Input: part model. Units: mm. Frame: model coordinates. A direction names the side the tool comes from. Coordinates: 2 decimals unless noted, no trailing zeros. Loops run counter-clockwise (first coordinate to the right, second up) from the corner with the lowest first, then second, coordinate; pieces in that order, holes last. Notation, with made-up numbers: (-0.75, 47) -> (7.25, 47) arc R22 ccw to (7.25, 72) -> close; hole circle Ø10 at (-1, 71). An arc over 180 degrees is marked (long way). Answer as a JSON object with one key per item and string values.
Autodesk Inventor part; units mm, degrees
ref_plane "YZ Plane" through (0, 0, 0) normal (1, 0, 0) x (0, 1, 0)
ref_plane "XZ Plane" through (0, 0, 0) normal (0, 1, 0) x (-1, 0, 0)
ref_plane "XY Plane" through (0, 0, 0) normal (0, 0, 1) x (1, 0, 0)
sketch "Sketch1" plane through (0, 0, 0) normal (0, 0, 1) x (1, 0, 0)
  circle A0 centre (0, 0) radius 120
  circle A1 centre (0, 0) radius 18
  dimension "d0" = 240
  dimension "d1" = 36
extrude "Extrusion1" add sketch "Sketch1" along normal blind 15
sketch "Sketch2" plane through (0, 0, 15) normal (0, 0, 1) x (1, 0, 0)
  circle A0 centre (79.5, 0) radius 23.5
  circle A1 centre (0, 79.5) radius 23.5
  circle A2 centre (-79.5, 0) radius 23.5
  circle A3 centre (0, -79.5) radius 23.5
  point P0 (0, 0)
  dimension "d5" = 47
  dimension "d7" = 47
  dimension "d8" = 47
  dimension "d9" = 47
extrude "Extrusion2" cut sketch "Sketch2" against normal blind 12
sketch "Sketch3" plane through (0, 0, 15) normal (0, 0, 1) x (1, 0, 0)
  circle A0 centre (0, 0) radius 21
  dimension "d12" = 42
extrude "Extrusion3" cut sketch "Sketch3" against normal blind 12
sketch "Sketch4" plane through (0, 0, 15) normal (0, 0, 1) x (1, 0, 0)
  circle A0 centre (0, 0) radius 18
  circle A1 centre (0, 0) radius 119
  circle A2 centre (0, 0) radius 120
  dimension "d15" = 238
  dimension "d16" = 240
extrude "Extrusion4" cut sketch "Sketch4" against normal blind 2 contours A2
sketch "Sketch5" plane through (0, 0, 15) normal (0, 0, 1) x (1, 0, 0)
  circle A0 centre (0, 0) radius 21
  line L0 (0, 0) -> (0, 113.556) construction
  circle A1 centre (0, 113.556) radius 2.5
  circle A2 centre (0, 0) radius 18
  circle A3 centre (0, 0) radius 113.556
  circle A4 centre (-66.7465, 91.8687) radius 2.5
  circle A5 centre (-107.9982, 35.0907) radius 2.5
  circle A6 centre (-107.9982, -35.0907) radius 2.5
  circle A7 centre (-66.7465, -91.8687) radius 2.5
  circle A8 centre (0, -113.556) radius 2.5
  circle A9 centre (66.7465, -91.8687) radius 2.5
  circle A10 centre (107.9982, -35.0907) radius 2.5
  circle A11 centre (107.9982, 35.0907) radius 2.5
  circle A12 centre (66.7465, 91.8687) radius 2.5
  dimension "d19" = 113.556
  dimension "d20" = 5
  dimension "d24" = 360
extrude "Extrusion5" cut sketch "Sketch5" against normal blind 15 contours A1 A3 | A3 A1 | A4 A3 | A3 A4 | A12 A3 | A3 A12 | A5 A3 | A3 A5 | A11 A3 | A3 A11 | A6 A3 | A3 A6 | A10 A3 | A3 A10 | A7 A3 | A3 A7 | A9 A3 | A3 A9 | A8 A3 | A3 A8
sketch "Sketch7" plane through (0, 0, 0) normal (0, 0, -1) x (-1, 0, 0)
  circle A0 centre (0, 113.556) radius 2.5
  circle A1 centre (0, 113.556) radius 6.12
  circle A2 centre (0, 0) radius 113.556 construction
  circle A3 centre (0, 0) radius 113.556 construction
  circle A4 centre (-66.7465, 91.8687) radius 6.12
  circle A5 centre (0, 0) radius 113.556 construction
  circle A6 centre (-107.9982, 35.0907) radius 6.12
  circle A7 centre (0, 0) radius 113.556 construction
  circle A8 centre (-107.9982, -35.0907) radius 6.12
  circle A9 centre (0, 0) radius 113.556 construction
  circle A10 centre (-66.7465, -91.8687) radius 6.12
  circle A11 centre (0, 0) radius 113.556 construction
  circle A12 centre (0, -113.556) radius 6.12
  circle A13 centre (0, 0) radius 113.556 construction
  circle A14 centre (66.7465, -91.8687) radius 6.12
  circle A15 centre (0, 0) radius 113.556 construction
  circle A16 centre (107.9982, -35.0907) radius 6.12
  circle A17 centre (0, 0) radius 113.556 construction
  circle A18 centre (107.9982, 35.0907) radius 6.12
  circle A19 centre (0, 0) radius 113.556 construction
  circle A20 centre (66.7465, 91.8687) radius 6.12
  dimension "d28" = 12.24
  dimension "d31" = 360
extrude "Extrusion6" cut sketch "Sketch7" against normal blind 2 contours A0 | A1 | A4 | A6 | A8 | A10 | A12 | A14 | A16 | A18 | A20
properties part number "Tampa_Superior"
1. Mould query, pull axis X, two halves, no side actions, for faces 3 (the face through (102.345, -37.435, 0.986)), 4 (the face through (-2, -25, 15)), 5 (the face through (-113.652, -37.435, 0.986)), 6 (the face through (63.974, 100.341, 14.014)). Classes: pulls with the +X half, pulls with the -X half, needs draft (parallel to the pull), parting line crosses it, or undercut.
Reply:
{"face 3": "undercut", "face 4": "needs draft", "face 5": "undercut", "face 6": "parting line crosses it"}
2. Pin query (flat end, axial travel): P1, Ø6, axis at x = 77, z = 10, coming from the -Y side; P2, Ø4, axis at x = 108, y = 35.09, coming from the +Z side; P3, Ø1, axis at x = -15, z = 2.5, coming from the +Y side; P4, Ø7.5, axis at x = 0, y = 113.556, coming from the -Z side. Return the tip coordinate at first contact, or that it passes through.
Reply:
{"P1": "stops at y = -94.47", "P2": "passes through", "P3": "stops at y = 119.12", "P4": "stops at z = 2"}
3. Section query D-D (z = 10.75). Count the separate pieces of the cut face and the enclosed holes in it, plus the area to 3 significant figures.
Reply:
{"separate pieces": "1", "enclosed holes": "15", "area": "36,700 mm2"}
4. Access query for faces 1 (the face through (105, -35, 2)), 2 (the face through (56.023, 1.033, 9.084)). Directions: +Z, -Z, +X, -X, +Y, -Y. A direction counts if a zero-diameter tool reaches every point of the face in a straight line with its end or side. Return the directions, or none.
Reply:
{"face 1": "-Z", "face 2": "+Z"}
5. Section query B-B (y = 79.5). Return loops of the section in (x, z), plus the area to 3 significant figures.
Reply:
{"outline": "(-89.89, 0) -> (89.89, 0) -> (89.89, 13) -> (88.55, 13) -> (88.55, 15) -> (23.5, 15) -> (23.5, 3) -> (-23.5, 3) -> (-23.5, 15) -> (-88.55, 15) -> (-88.55, 13) -> (-89.89, 13) -> close", "area": "2,130 mm2"}
6. Line query: line 1 along Y through (x, z) = (0, 1.35); line 2 along Y through (x, z) = (0, 5.5); line 3 along Y through (x, z) = (66, 6.25). Output: solid intervals per line, ascending.
Reply:
{"line 1": "y = -120 to -119.68, -107.44 to -18, 18 to 107.44, 119.68 to 120", "line 2": "y = -120 to -116.06, -111.06 to -103, -56 to -21, 21 to 56, 103 to 111.06, 116.06 to 120", "line 3": "y = -100.22 to -94.25, -89.48 to -19.24, 19.24 to 89.48, 94.25 to 100.22"}
7. Section query A-A (y = 0). Return loops of the section in (x, z), plus the area to 3 significant figures.
Reply:
{"outline": "(-120, 0) -> (-18, 0) -> (-18, 3) -> (-21, 3) -> (-21, 15) -> (-56, 15) -> (-56, 3) -> (-103, 3) -> (-103, 15) -> (-119, 15) -> (-119, 13) -> (-120, 13) -> close; (18, 0) -> (120, 0) -> (120, 13) -> (119, 13) -> (119, 15) -> (103, 15) -> (103, 3) -> (56, 3) -> (56, 15) -> (21, 15) -> (21, 3) -> (18, 3) -> close", "area": "1,860 mm2"}
